The listing builds one solid part. Answer for the finished solid, in the listing's coordinates (mm). A direction names the side the tool comes from. Coordinates: 2 decimals unless noted, no trailing zeros. Write each loop counter-clockwise with the first axis right and the second up, starting at its lowest first coordinate (ties: lowest second). Pieces come first, ordered by that corner, then holes.
(1) The part is cut by section D-D on z = -20. Determine the outline of the cut face in (x, y), plus the area to 3 significant figures.
(2) For a pull along Z with two mould halves and no side action, classify faces 4 (the cylindrical face through (9.352, 1.521, -8.474)), 5 (the flat face through (18, 1, 0)), 6 (the flat face through (18, 1, -30)), 7 (the flat face through (73, 1, -15)) as +Z half, -Z half, draft (parallel to the pull), parting line (faces both ways), or undercut.
(3) Straight lines are drawn through the part: line 1 (X direction, y = 1.15, z = -15); line 2 (X direction, y = 1.8, z = -7); line 3 (Z direction, x = 17, y = 2.3). For each, find the intervals that lie inside material, in ascending order.
(4) Given P1, Ø0.9, axis at x = 18, y = 2, coming from the +Z side; P2, Ø3, axis at x = 23, z = -7, coming from the +Y side; P3, Ø1, axis at x = 27, y = 1.5, coming from the -Z side; P4, Ø0.9, axis at y = 2, z = -34.5, coming from the -X side, each flat-ended and moving along its own axis, determine where each tip first touches the part or whether it passes through.
(5) The part is cut by section C-C on y = 1.1. Give the number of separate pieces and of enclosed holes in the cut face, plus the area to 3 significant figures.
(6) Which of the six approach directions +Z, -Z, +X, -X, +Y, -Y give full straight-line access (tool end or side, diameter ignored) to faces 1 (the flat face through (45, 3, -15)), 2 (the flat face through (36, 1, 8)), 3 (the flat face through (36, 1, -37))?
(7) The part is cut by section A-A on x = 8. Determine the outline of the cut face in (y, z), plus the area to 3 significant figures.
(8) The part is cut by section B-B on x = 49.5. Determine the outline of the cut face in (y, z).
from build123d import *

# Parameters (mm, degrees)
EXTRUDE_1_DEPTH     = 3
SKETCH_2_R          = 2
SKETCH_2_R_2        = 6
CUT_EXTRUDE_1_DEPTH = 3
SKETCH_3_R          = 1.25
CUT_EXTRUDE_2_DEPTH = 3


with BuildPart() as part:
    # 草图1 → 凸台-拉伸1 (new body)
    with BuildSketch(Plane(origin=(0, 0, 0), x_dir=(1, 0, 0), z_dir=(0, 1, 0))):
        Polygon((0, 0), (0, 30), (36, 30), (36, 45), (73, 45), (73, -15), (36, -15), (36, 0), align=None)
    extrude(amount=EXTRUDE_1_DEPTH)

    # 草图2 → 切除-拉伸1 (cut)
    with BuildSketch(Plane(origin=(0, 3, 0), x_dir=(1, 0, 0), z_dir=(0, 1, 0))):
        with Locations(Location((8, 23, 0), (0, 0, 270))):
            Circle(SKETCH_2_R)
        with Locations(Location((23, 23, 0), (0, 0, 270))):
            Circle(SKETCH_2_R)
        with Locations(Location((8, 7, 0), (0, 0, 270))):
            Circle(SKETCH_2_R)
        with Locations(Location((23, 7, 0), (0, 0, 270))):
            Circle(SKETCH_2_R)
        with Locations(Location((59, 15, 0), (0, 0, 270))):
            Circle(SKETCH_2_R_2)
    extrude(amount=-CUT_EXTRUDE_1_DEPTH, mode=Mode.SUBTRACT)

    # 草图3 → 切除-拉伸2 (cut)
    with BuildSketch(Plane(origin=(0, 3, 0), x_dir=(1, 0, 0), z_dir=(0, 1, 0))):
        with Locations(Location((63.75, 23.227241336, 0), (0, 0, 270))):
            Circle(SKETCH_3_R)
        with Locations(Location((63.75, 6.772758664, 0), (0, 0, 270))):
            Circle(SKETCH_3_R)
        with Locations(Location((49.5, 15, 0), (0, 0, 270))):
            Circle(SKETCH_3_R)
    extrude(amount=-CUT_EXTRUDE_2_DEPTH, mode=Mode.SUBTRACT)


solid = part.part
Model answer:
1. outline: (0, 0) - (55.68, 0) - (55.68, 3) - (0, 3) - close; (62.32, 0) - (73, 0) - (73, 3) - (62.32, 3) - close
1. area: 199 mm2
2. face 4: undercut
2. face 5: +Z half
2. face 6: -Z half
2. face 7: draft
3. line 1: x = 0 to 48.25, 50.75 to 53, 65 to 73
3. line 2: x = 0 to 6, 10 to 21, 25 to 62.52, 64.98 to 73
3. line 3: z = -30 to 0
4. P1: stops at z = 0
4. P2: passes through
4. P3: stops at z = -30
4. P4: stops at x = 36
5. separate pieces: 1
5. enclosed holes: 8
5. area: 3,120 mm2
6. face 1: +Z, -Z, +X, -X, +Y
6. face 2: +Z, -X, +Y, -Y
6. face 3: -Z, -X, +Y, -Y
7. outline: (0, -30) - (3, -30) - (3, -25) - (0, -25) - close; (0, -21) - (3, -21) - (3, -9) - (0, -9) - close; (0, -5) - (3, -5) - (3, 0) - (0, 0) - close
7. area: 66.0 mm2
8. outline: (0, -45) - (3, -45) - (3, -16.25) - (0, -16.25) - close; (0, -13.75) - (3, -13.75) - (3, 15) - (0, 15) - close
